Geometry: final body of the model. Coordinates: model frame, mm. A direction names the side the tool comes from. Give positions to 0.01 mm unless a question says otherwise; leave off trailing zeros. Write each loop counter-clockwise with the first axis right and the second up, starting at its lowest first coordinate (ties: lowest second). Pieces come first, ordered by that corner, then holes. Notation, with made-up numbers: (27.5, -8.75) -> (74.5, -8.75) arc R32 cw to (74.5, 25.25) -> close; hole circle Ø11 at (81, 74). An arc over 180 degrees is marked (long way). Answer as a JSON object with one key per item and string values. Group by question number.
(1) Section query D-D on z = -40.5. Output: boundary loops of the cut face in (x, y), plus the area to 3 significant figures.
(2) Section query B-B on x = 0. Output: boundary loops of the cut face in (y, z) (3 decimals), plus the area to 3 significant figures.
(3) Set-up query: faces 4 (the face through (-38.1, -13, 0)), 5 (the face through (-31.75, -13, 44)), 6 (the face through (51, -13, -6.35)). Return all of +Z, -Z, +X, -X, +Y, -Y with unobstructed straight access to the full face (end or side cutting, diameter ignored); none if empty.
(4) Contact query for flat-ended pins moving along their axis: pin 1 Ø7 at (x, y) = (48.5, -13.5) entering from +Z; pin 2 Ø2 at (x, y) = (37.5, -13) entering from -Z; pin 3 Ø5 at (y, z) = (6.5, -27.5) entering from -X; pin 4 Ø1 at (x, z) = (-6, 12.5) entering from +Y. Output: stop coordinate, or through.
(5) Draft query along X for faces 1 (the face through (0, -13, -38.1)), 2 (the face through (60.494, -12.522, 19.306)), 3 (the face through (50, -13, 6.35)). Return one class per face: +X half, -X half, draft (parallel to the pull), parting line (faces both ways), or undercut.
(6) Material intervals for probe 1 along Z at (x, y) = (-52, -7); probe 2 along Z at (x, y) = (0, -18.5) (3 decimals); probe 3 along Y at (x, z) = (-30, -34.5), sorted ascending.
(7) Section query A-A on z = 0. Output: boundary loops of the cut face in (x, y) (3 decimals).
from build123d import *

# Parameters (mm, degrees)
F0_R     = 28.575
F0_R_2   = 15.875
F1_DEPTH = 25.4
F2_DEPTH = 19.05


with BuildPart() as f1:
    # F0 (on Front) → F1 (new body)
    with BuildSketch(Plane.XZ):
        with BuildLine():
            Line((38.1, 6.35), (63.181702, 6.35))
            ThreePointArc((63.181702, 6.35), (60.436597, 19.485066), (54.992613, 31.75))
            Line((54.992613, 31.75), (31.75, 31.75))
            Line((31.75, 31.75), (31.75, 54.992613))
            ThreePointArc((31.75, 54.992613), (19.485066, 60.436597), (6.35, 63.181702))
            Line((6.35, 63.181702), (6.35, 38.1))
            Line((6.35, 38.1), (0, 38.1))
            Line((0, 38.1), (-6.35, 38.1))
            Line((-6.35, 38.1), (-6.35, 63.181702))
            ThreePointArc((-6.35, 63.181702), (-19.485066, 60.436597), (-31.75, 54.992613))
            Line((-31.75, 54.992613), (-31.75, 31.75))
            Line((-31.75, 31.75), (-54.992613, 31.75))
            ThreePointArc((-54.992613, 31.75), (-60.436597, 19.485066), (-63.181702, 6.35))
            Line((-63.181702, 6.35), (-38.1, 6.35))
            Line((-38.1, 6.35), (-38.1, 0))
            Line((-38.1, 0), (-38.1, -6.35))
            Line((-38.1, -6.35), (-63.181702, -6.35))
            ThreePointArc((-63.181702, -6.35), (-60.436597, -19.485066), (-54.992613, -31.75))
            Line((-54.992613, -31.75), (-31.75, -31.75))
            Line((-31.75, -31.75), (-31.75, -54.992613))
            ThreePointArc((-31.75, -54.992613), (-19.485066, -60.436597), (-6.35, -63.181702))
            Line((-6.35, -63.181702), (-6.35, -38.1))
            Line((-6.35, -38.1), (0, -38.1))
            Line((0, -38.1), (6.35, -38.1))
            Line((6.35, -38.1), (6.35, -63.181702))
            ThreePointArc((6.35, -63.181702), (19.485066, -60.436597), (31.75, -54.992613))
            Line((31.75, -54.992613), (31.75, -31.75))
            Line((31.75, -31.75), (54.992613, -31.75))
            ThreePointArc((54.992613, -31.75), (60.436597, -19.485066), (63.181702, -6.35))
            Line((63.181702, -6.35), (38.1, -6.35))
            Line((38.1, -6.35), (38.1, 0))
            Line((38.1, 0), (38.1, 6.35))
        make_face()
        Circle(F0_R, mode=Mode.SUBTRACT)
        Circle(F0_R)
        Circle(F0_R_2, mode=Mode.SUBTRACT)
    extrude(amount=F1_DEPTH)

    # F0 (on Front) → F2 (join)
    with BuildSketch(Plane.XZ):
        Circle(F0_R)
        Circle(F0_R_2, mode=Mode.SUBTRACT)
    extrude(amount=-F2_DEPTH)


solid = f1.part
Answer list:
{
 "1": {"outline": "(-31.75, -25.4) -> (-6.35, -25.4) -> (-6.35, 0) -> (-31.75, 0) -> close; (6.35, -25.4) -> (31.75, -25.4) -> (31.75, 0) -> (6.35, 0) -> close", "area": "1,290 mm2"},
 "2": {"outline": "(-25.4, -38.1) -> (0, -38.1) -> (0, -28.575) -> (19.05, -28.575) -> (19.05, -15.875) -> (-25.4, -15.875) -> close; (-25.4, 15.875) -> (19.05, 15.875) -> (19.05, 28.575) -> (0, 28.575) -> (0, 38.1) -> (-25.4, 38.1) -> close", "area": "1,610 mm2"},
 "3": {"face 4": "-X, +Y, -Y", "face 5": "+Z, -X, +Y, -Y", "face 6": "+X, +Y, -Y"},
 "4": {"pin 1": "z = 31.75", "pin 2": "z = -31.75", "pin 3": "x = -13.84", "pin 4": "through"},
 "5": {"face 1": "undercut", "face 2": "+X half", "face 3": "draft"},
 "6": {"probe 1": "-31.75 to -6.35, 6.35 to 31.75", "probe 2": "-38.1 to -15.875, 15.875 to 38.1", "probe 3": "-25.4 to 0"},
 "7": {"outline": "(-38.1, -25.4) -> (-15.875, -25.4) -> (-15.875, 19.05) -> (-28.575, 19.05) -> (-28.575, 0) -> (-38.1, 0) -> close; (15.875, -25.4) -> (38.1, -25.4) -> (38.1, 0) -> (28.575, 0) -> (28.575, 19.05) -> (15.875, 19.05) -> close"}
}
